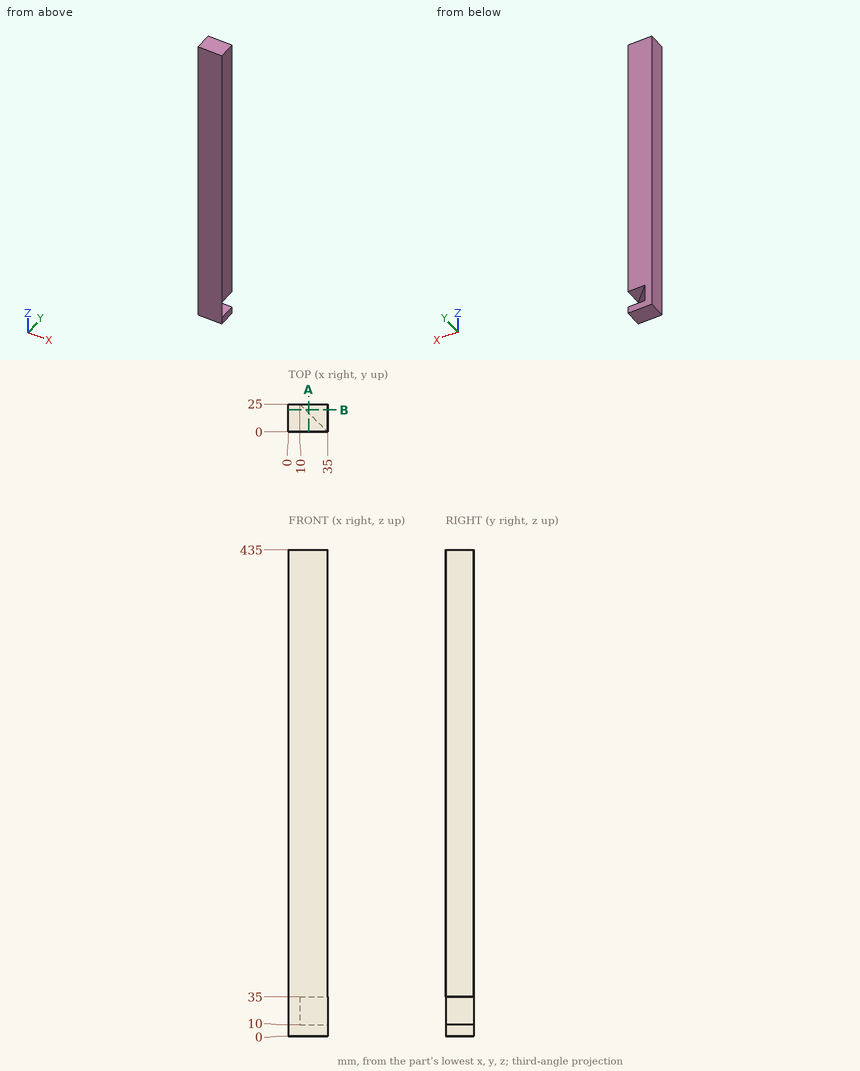
Print and shaded views of the part. All mm, measured from the part's lowest x, y and z. Give positions to 0.01 mm unless a question says otherwise; leave off trailing zeros. Write each loop counter-clockwise with the first axis right and the second up, starting at its lowest first coordinate (ties: lowest second). Pieces come first, ordered by that corner, then holes. Notation, with made-up numbers: (18.25, -26) - (22.25, -26) arc R19 ccw to (22.25, -13) - close; hole circle Ø7 at (48.5, 26). An arc over 180 degrees is marked (long way). One line per question, with ' | ' between items. Start each with the question number.
(1) Pin check, flat tip, straight feed: P1, Ø6, axis at x = 22, y = 14, coming from the -Z side. Stop position of the tip, or through.
(2) Slice it at A-A on x = 18. Write the cut outline in (y, z), plus the area to 3 significant figures.
(3) Slice it at B-B on y = 19.75. Write the cut outline in (x, z), plus the area to 3 significant figures.
(4) Wall check: line 1 along Z through (x, y) = (22.5, 15.75); line 2 along Y through (x, z) = (13, 25.5); line 3 along X through (y, z) = (17.5, 24). Give the ranges that are in metal, low to high. Write a range as from..to.
Results below:
1) P1: z = 0
2) outline: (0, 0) - (25, 0) - (25, 10) - (17, 10) - (17, 35) - (25, 35) - (25, 435) - (0, 435) - close | area: 10,700 mm^2
3) outline: (0, 0) - (35, 0) - (35, 10) - (15.25, 10) - (15.25, 35) - (35, 35) - (35, 435) - (0, 435) - close | area: 14,700 mm^2
4) line 1: 0..10, 35..435 | line 2: 0..22 | line 3: 0..17.5
